```python
from build123d import *

# Parameters (mm, degrees)
F0_W     = 50
F0_H     = 45.5
F0_R     = 3.2
F0_R_2   = 5
F0_R_3   = 11.35
F1_DEPTH = 4
F0_R_4   = 1.7
F2_DEPTH = 1
F3_DEPTH = 3
F4_SIZE  = 8


# Not quite as in the source:
# - a feature names something its author has since deleted; it is built from what else it names


with BuildPart() as f1:
    # F0 (on Top) → F1 (new body)
    with BuildSketch(Plane.XY):
        with Locations((0, -1.75)):
            Rectangle(F0_W, F0_H)
        with Locations((-15.5, -15.5)):
            Circle(F0_R, mode=Mode.SUBTRACT)
        with Locations((-6.4, -15.4509711824)):
            Circle(F0_R_2, mode=Mode.SUBTRACT)
        with Locations((-15.4509711824, -6.4)):
            Circle(F0_R_2, mode=Mode.SUBTRACT)
        with Locations((6.4, -15.4509711824)):
            Circle(F0_R_2, mode=Mode.SUBTRACT)
        with Locations((15.5, -15.5)):
            Circle(F0_R, mode=Mode.SUBTRACT)
        with Locations((15.4509711824, -6.4)):
            Circle(F0_R_2, mode=Mode.SUBTRACT)
        with Locations((-15.4509711824, 6.4)):
            Circle(F0_R_2, mode=Mode.SUBTRACT)
        with Locations((-15.5, 15.5)):
            Circle(F0_R, mode=Mode.SUBTRACT)
        with Locations((-6.4, 15.4509711824)):
            Circle(F0_R_2, mode=Mode.SUBTRACT)
        Circle(F0_R_3, mode=Mode.SUBTRACT)
        with Locations((15.4509711824, 6.4)):
            Circle(F0_R_2, mode=Mode.SUBTRACT)
        with Locations((6.4, 15.4509711824)):
            Circle(F0_R_2, mode=Mode.SUBTRACT)
        with Locations((15.5, 15.5)):
            Circle(F0_R, mode=Mode.SUBTRACT)
        with Locations((-15.4509711824, -6.4)):
            Circle(F0_R_2)
        with Locations((-6.4, -15.4509711824)):
            Circle(F0_R_2)
        with Locations((6.4, -15.4509711824)):
            Circle(F0_R_2)
        with Locations((15.4509711824, -6.4)):
            Circle(F0_R_2)
        with Locations((15.4509711824, 6.4)):
            Circle(F0_R_2)
        with Locations((6.4, 15.4509711824)):
            Circle(F0_R_2)
        with Locations((-6.4, 15.4509711824)):
            Circle(F0_R_2)
        with Locations((-15.4509711824, 6.4)):
            Circle(F0_R_2)
    extrude(amount=F1_DEPTH)

    # F0 (on Top) → F2 (join)
    with BuildSketch(Plane.XY):
        with Locations((-15.5, 15.5)):
            Circle(F0_R)
        with Locations((-15.5, 15.5)):
            Circle(F0_R_4, mode=Mode.SUBTRACT)
        with Locations((15.5, 15.5)):
            Circle(F0_R)
        with Locations((15.5, 15.5)):
            Circle(F0_R_4, mode=Mode.SUBTRACT)
        with Locations((15.5, -15.5)):
            Circle(F0_R)
        with Locations((15.5, -15.5)):
            Circle(F0_R_4, mode=Mode.SUBTRACT)
        with Locations((-15.5, -15.5)):
            Circle(F0_R)
        with Locations((-15.5, -15.5)):
            Circle(F0_R_4, mode=Mode.SUBTRACT)
    extrude(amount=F2_DEPTH)

    # F0 (on Top) → F3 (cut)
    with BuildSketch(Plane.XY):
        with Locations((-15.4509711824, -6.4)):
            Circle(F0_R_2)
        with Locations((-6.4, -15.4509711824)):
            Circle(F0_R_2)
        with Locations((6.4, -15.4509711824)):
            Circle(F0_R_2)
        with Locations((15.4509711824, -6.4)):
            Circle(F0_R_2)
        with Locations((15.4509711824, 6.4)):
            Circle(F0_R_2)
        with Locations((6.4, 15.4509711824)):
            Circle(F0_R_2)
        with Locations((-6.4, 15.4509711824)):
            Circle(F0_R_2)
        with Locations((-15.4509711824, 6.4)):
            Circle(F0_R_2)
    extrude(amount=F3_DEPTH, mode=Mode.SUBTRACT)

    # F4
    f4_edges = [f1.edges().sort_by_distance(p)[0] for p in [
        (25, 21, 2),
        (-25, 21, 2),
        (25, -24.5, 2),
        (-25, -24.5, 2),
    ]]
    chamfer(f4_edges, length=F4_SIZE)


solid = f1.part
```
Here's how the part is built. I have some questions about the finished solid (model axes, mm). A direction names the side the tool comes from. Coordinates: 2 decimals unless noted, no trailing zeros. Write each loop counter-clockwise with the first axis right and the second up, starting at its lowest first coordinate (ties: lowest second). Pieces come first, ordered by that corner, then holes. Notation, with made-up numbers: M 13.5,-15.75 L 62.5,-15.75 A13 ccw 62.5,5.25 Z; hole C 53,54 d5. An arc over 180 degrees is marked long. Answer as CSV lines item,"result". Start each with the question number.
Q1. Suppose I cut it at D-D, the plane x = 4. List the corners of the cut face in (y, z) for me, then the cut area to 3 significant figures.
Q2. Suppose I cut it at B-B, the plane x = -15.5. List the corners of the cut face in (y, z) for me, then the cut area to 3 significant figures.
Q3. If we mould it in two halves opening along X, with no side actions, what happens to faces 4 (the flat face through (-25, -2, 2)), 5 (the cylindrical face through (9.088, 19.667, 1.479)), 6 (the flat face through (0, -12, 4))? For each: pulls with the +X half, pulls with the -X half, needs draft (parallel to the pull), parting line crosses it, or undercut.
Q4. I need wall thicknesses on probe 1 along Y at (x, z) = (15.5, 0.55); probe 2 along Y at (x, z) = (15.5, 2.05); probe 3 along Y at (x, z) = (-6.5, 1.1). Which ranges of each line are inside material? Lowest first, please. Write a range as [from, to].
Q5. Suppose I cut it at A-A, the plane y = 0. List the corners of the cut face in (x, z) for me.
Q6. For faces 1 (the flat face through (-16, 6, 3)), 2 (the cylindrical face through (14.806, -18.624, 2.479)), 3 (the flat face through (-21, 17, 2)), which set-ups out of +Z, -Z, +X, -X, +Y, -Y let a thin tool reach every point of the face, with its end or its side?
Q7. Will these pins go through, and if not, where does the flat tip stop? pin 1 Ø3 at (x, y) = (14, -5) entering from -Z; pin 2 Ø5 at (x, y) = (-16.5, -14) entering from +Z; pin 3 Ø6 at (x, y) = (-15.5, -15.5) entering from +Z; pin 4 Ø2.5 at (x, y) = (-15.5, -15.5) entering from -Z.
Q8. Suppose I cut it at C-C, the plane y = 16.5. List the corners of the cut face in (x, z) for me, then the cut area to 3 significant figures.
Entries:
1,outline,"M -24.5,0 L -19.84,0 L -19.84,3 L -11.06,3 L -11.06,0 L -10.62,0 L -10.62,4 L -24.5,4 Z; M 10.62,0 L 11.06,0 L 11.06,3 L 19.84,3 L 19.84,0 L 21,0 L 21,4 L 10.62,4 Z"
1,area,"44.4 mm²"
2,outline,"M -24.5,0 L -17.2,0 L -17.2,1 L -18.7,1 L -18.7,4 L -24.5,4 Z; M -13.8,0 L -11.4,0 L -11.4,3 L -1.4,3 L -1.4,0 L 1.4,0 L 1.4,3 L 11.4,3 L 11.4,0 L 13.8,0 L 13.8,1 L 12.3,1 L 12.3,4 L -12.3,4 L -12.3,1 L -13.8,1 Z; M 17.2,0 L 21,0 L 21,4 L 18.7,4 L 18.7,1 L 17.2,1 Z"
2,area,"76.8 mm²"
3,face 4,"pulls with the -X half"
3,face 5,"undercut"
3,face 6,"needs draft"
4,probe 1,"y = [-24.5, -17.2], [-13.8, -11.4], [-1.4, 1.4], [11.4, 13.8], [17.2, 21]"
4,probe 2,"y = [-24.5, -18.7], [-12.3, -11.4], [-1.4, 1.4], [11.4, 12.3], [18.7, 21]"
4,probe 3,"y = [-24.5, -20.45], [-10.45, -9.3], [9.3, 10.45], [20.45, 21]"
5,outline,"M -25,0 L -11.35,0 L -11.35,4 L -25,4 Z; M 11.35,0 L 25,0 L 25,4 L 11.35,4 Z"
6,face 1,"-Z"
6,face 2,"+Z"
6,face 3,"+Z, -Z, -X, +Y"
7,pin 1,"stops at z = 3"
7,pin 2,"stops at z = 4"
7,pin 3,"stops at z = 1"
7,pin 4,"passes through"
8,outline,"M -21.5,0 L -16.87,0 L -16.87,1 L -18.54,1 L -18.54,4 L -21.5,4 Z; M -14.13,0 L -11.29,0 L -11.29,3 L -1.51,3 L -1.51,0 L 1.51,0 L 1.51,3 L 11.29,3 L 11.29,0 L 14.13,0 L 14.13,1 L 12.46,1 L 12.46,4 L -12.46,4 L -12.46,1 L -14.13,1 Z; M 16.87,0 L 21.5,0 L 21.5,4 L 18.54,4 L 18.54,1 L 16.87,1 Z"
8,area,"71.4 mm²"
